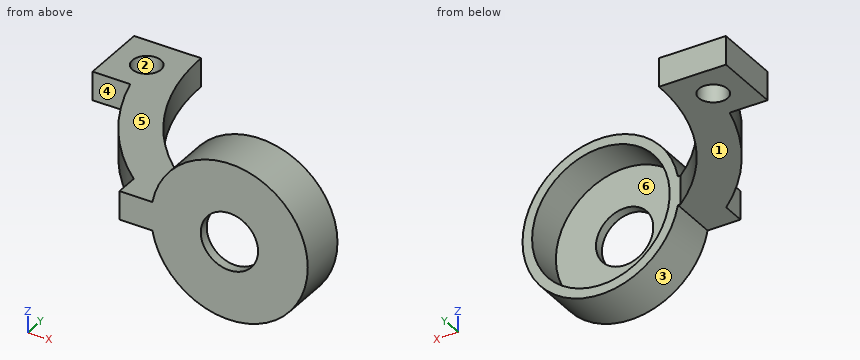
```python
from build123d import *

# Parameters (mm, degrees)
SKETCH4_R           = 0.75
BOSS_EXTRUDE1_DEPTH = 1.5
BOSS_EXTRUDE2_REACH = 19.027
SKETCH3_W           = 2.850862197
SKETCH3_H           = 1.5
CUT_EXTRUDE1_START  = -2
SKETCH5_R           = 3.6
CUT_EXTRUDE1_DEPTH  = 2


with BuildPart() as part:
    # Sketch1 → Revolve1 (revolve)
    with BuildSketch(Plane.XY):
        Polygon((4.1, 0), (4.1, 2.5), (3.6, 2.5), (3.6, 0.5), (1.5, 0.5), (1.5, 0), align=None)
    revolve(axis=Axis((0, 0, 0), (0, 1, 0)))

    # Boss-Extrude2: up to this face of the body (flat: up to its plane)
    boss_extrude2_end = Plane(part.part.faces().sort_by_distance((-3.984034488, 2.5, 0))[0])
    # Sketch3 → Boss-Extrude2 (add, up to the picked face)
    with BuildSketch(Plane.XZ, mode=Mode.PRIVATE) as boss_extrude2_sk1:
        with Locations((-4.324568902, 0)):
            Rectangle(SKETCH3_W, SKETCH3_H)
    boss_extrude2_tool1 = split(extrude(boss_extrude2_sk1.sketch, amount=-BOSS_EXTRUDE2_REACH, mode=Mode.PRIVATE), bisect_by=boss_extrude2_end, keep=Keep.BOTH, mode=Mode.PRIVATE)


with BuildPart() as body_2:
    # Sketch4 → Boss-Extrude1 (new body)
    with BuildSketch(Plane.XY.offset(-0.75)):
        with BuildLine():
            Line((-8.530818775, 11.33), (-12.030818775, 11.33))
            Line((-12.030818775, 11.33), (-12.030818775, 7.83))
            Line((-12.030818775, 7.83), (-10.055529403, 7.83))
            ThreePointArc((-10.055529403, 7.83), (-7.808057008, 3.326468933), (-4.030818775, 0))
            Line((-4.030818775, 0), (-4.172844356, 2.5))
            ThreePointArc((-4.172844356, 2.5), (-7.382007257, 6.406565197), (-8.530818775, 11.33))
        make_face()
        with Locations((-10.280818775, 9.58)):
            Circle(SKETCH4_R, mode=Mode.SUBTRACT)
    extrude(amount=BOSS_EXTRUDE1_DEPTH)


with BuildPart() as part_1:
    add(part.part)

    add(body_2.part)  # Boss-Extrude2 merges body 2
    add(boss_extrude2_tool1.solids().sort_by(Axis((-4.324569, 0, 0), (0, 1, 0)))[0])

    # Sketch5 → Cut-Extrude1 (cut)
    with BuildSketch(Plane(origin=(0, 2.5, 0), x_dir=(1, 0, 0), z_dir=(0, 1, 0)).offset(CUT_EXTRUDE1_START)):
        Circle(SKETCH5_R)
    extrude(amount=CUT_EXTRUDE1_DEPTH, mode=Mode.SUBTRACT)


solid = part_1.part
```
Verification items for the finished model (mm, model axes). Face numbers are marked on the shaded views. A direction names the side the tool comes from. Coordinates: 2 decimals unless noted, no trailing zeros. Loops run counter-clockwise (first coordinate to the right, second up) from the corner with the lowest first, then second, coordinate; pieces in that order, holes last. Notation, with made-up numbers: (54.25, 69.5) -> (87.25, 69.5) arc R26 cw to (87.25, 83.5) -> close; hole circle Ø8 at (52.5, 28.5). An arc over 180 degrees is marked (long way). Answer in a Markdown table with one row per item. Add a question column.
1. Access from +Z, -Z, +X, -X, +Y, -Y to the whole of each face (thin tool, end or side, straight path). Record for the marked faces 4, 5 and 6.
2. Section check D-D, the plane z = -1. Enter the section's corners in (x, y).
3. Draft check along X on the marked faces 1, 2 and 3. Enter one of: +X half, -X half, draft (parallel to the pull), parting line (faces both ways), or undercut.
4. Section check A-A, the plane z = 0. Enter the section's corners in (x, y), then the cut area to 3 significant figures.
5. Depth check by flat-ended pin: P1, Ø4, axis at x = 0.5, z = -2.5, coming from the +Y side; P2, Ø6, axis at x = -7.5, y = 8, coming from the -Z side; P3, Ø2.5, axis at x = -2, z = 1, coming from the +Y side. Enter the tip coordinate at first touch or a pass-through.
6. Section check C-C, the plane y = 9.58. Enter the section's corners in (x, z), then the cut area to 3 significant figures.
7. Section check B-B, the plane x = 0. Enter the section's corners in (y, z), then the cut area to 3 significant figures.
8. Material ranges on probe 1 along X at (y, z) = (0.35, 0); probe 2 along Z at (x, y) = (0, 1.9); probe 3 along Z at (x, y) = (0, 0.3), recorded low to high. Write a range as [from, to].
Derived:
| question | item | result |
|---|---|---|
| 1 | face 4 | +Z, -Z, -X, -Y |
| 1 | face 5 | +Z, -X, +Y, -Y |
| 1 | face 6 | +Y |
| 2 | outline | (-3.98, 0) -> (-1.12, 0) -> (-1.12, 0.5) -> (-3.46, 0.5) -> (-3.46, 2.5) -> (-3.98, 2.5) -> close; (1.12, 0) -> (3.98, 0) -> (3.98, 2.5) -> (3.46, 2.5) -> (3.46, 0.5) -> (1.12, 0.5) -> close |
| 3 | face 1 | draft |
| 3 | face 2 | undercut |
| 3 | face 3 | parting line |
| 4 | outline | (-12.03, 7.83) -> (-10.06, 7.83) arc R13.12 ccw to (-5.75, 1.2) -> (-5.75, 0) -> (-1.5, 0) -> (-1.5, 0.5) -> (-3.6, 0.5) -> (-3.6, 2.5) -> (-4.17, 2.5) arc R11.12 cw to (-8.53, 11.33) -> (-12.03, 11.33) -> close; (1.5, 0) -> (4.1, 0) -> (4.1, 2.5) -> (3.6, 2.5) -> (3.6, 0.5) -> (1.5, 0.5) -> close; hole circle Ø1.5 at (-10.28, 9.58) |
| 4 | area | 33.5 mm² |
| 5 | P1 | stops at y = 2.5 |
| 5 | P2 | stops at z = -0.75 |
| 5 | P3 | stops at y = 0.5 |
| 6 | outline | (-12.03, -0.75) -> (-11.03, -0.75) -> (-11.03, 0.75) -> (-12.03, 0.75) -> close; (-9.53, -0.75) -> (-8.39, -0.75) -> (-8.39, 0.75) -> (-9.53, 0.75) -> close |
| 6 | area | 3.21 mm² |
| 7 | outline | (0, -4.1) -> (2.5, -4.1) -> (2.5, -3.6) -> (0.5, -3.6) -> (0.5, -1.5) -> (0, -1.5) -> close; (0, 1.5) -> (0.5, 1.5) -> (0.5, 3.6) -> (2.5, 3.6) -> (2.5, 4.1) -> (0, 4.1) -> close |
| 7 | area | 4.60 mm² |
| 8 | probe 1 | x = [-5.75, -1.5], [1.5, 4.1] |
| 8 | probe 2 | z = [-4.1, -3.6], [3.6, 4.1] |
| 8 | probe 3 | z = [-4.1, -1.5], [1.5, 4.1] |
